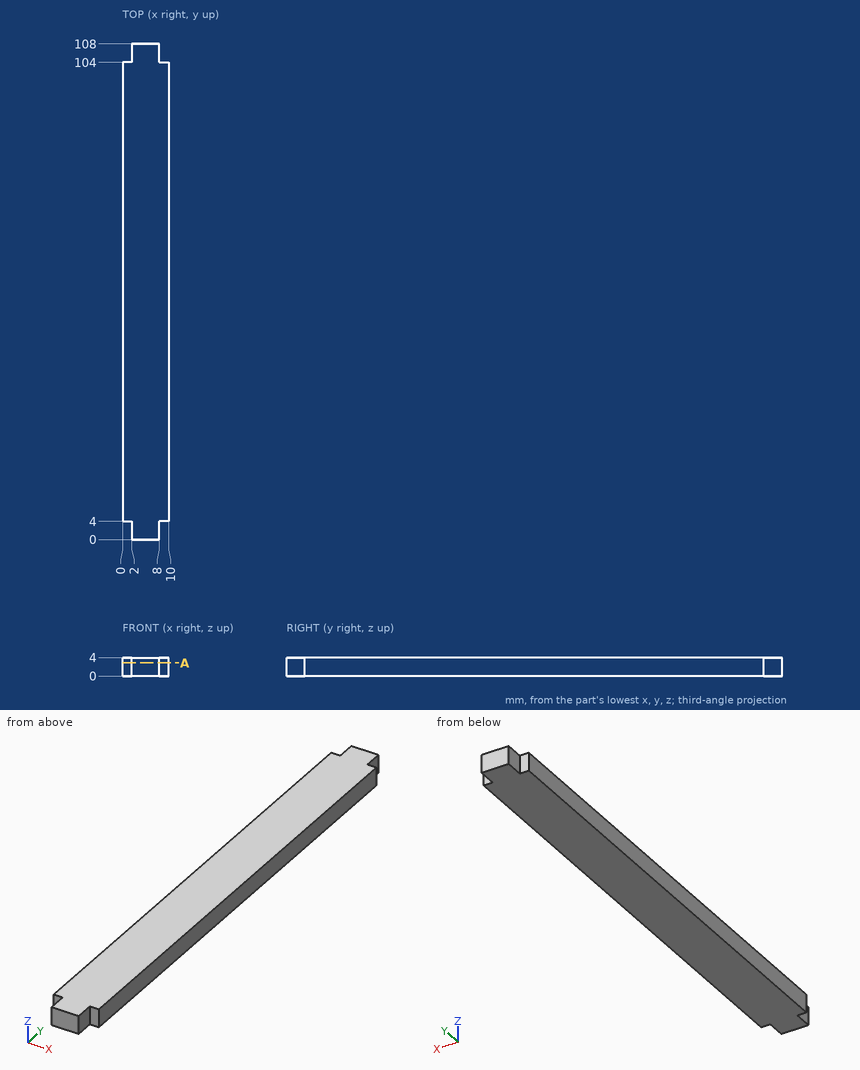
Answer from the drawing. Dimensions are ordinates in mm from the lowest x, y and z of the part. Give positions to 0.01 mm unless a question says otherwise; leave off trailing zeros. Write each loop counter-clockwise with the first axis right and the second up, starting at its lowest first coordinate (ties: lowest second). Pieces come first, ordered by that corner, then holes.
1) Find the intervals of material crossed by L1, parallel to Y at x = 8.5, z = 0.95, in increasing order.
2) Given P1, Ø0.6, axis at x = 1.5, z = 2.5, coming from the +Y side; P2, Ø2, axis at y = 2.5, z = 2.5, coming from the +X side; P3, Ø0.6, axis at x = 1.5, z = 3, coming from the -Y side, each flat-ended and moving along its own axis, determine where each tip first touches the part or whether it passes through.
3) Section A-A (z = 2.85) is taken. Write down the section's boundary in (x, y), and give its area (3 significant figures).
Response:
1. L1: y = 4 to 104
2. P1: stops at y = 104
2. P2: stops at x = 8
2. P3: stops at y = 4
3. outline: (0, 4) - (2, 4) - (2, 0) - (8, 0) - (8, 4) - (10, 4) - (10, 104) - (8, 104) - (8, 108) - (2, 108) - (2, 104) - (0, 104) - close
3. area: 1,050 mm2
